from build123d import *
from build123d.topology import SkipClean

# Parameters (mm, degrees)
SKETCH_2_R                = 22
EXTRUDE_1_DEPTH           = 5
SKETCH_5_W                = 7
SKETCH_5_H                = 15
EXTRUDE_2_DEPTH           = 5
HOLE_WIZARD_2_56_3_D      = 1.778
HOLE_WIZARD_2_56_3_DEPTH  = 15
HOLE_WIZARD_2_56_3_TIP    = 0.534165
SKETCH_13_R               = 20.05
CUT_EXTRUDE_2_DEPTH       = 4
SKETCH_14_R               = 19
CUT_EXTRUDE_3_DEPTH       = 2
CUT_EXTRUDE_4_DEPTH       = 38.016888
EXTRUDE_3_REACH           = 58.225
EXTRUDE_3_END_RADIUS      = 22
SKETCH_16_W               = 18.5
SKETCH_16_H               = 5
FILLET_1_R                = 2
CHAMFER_1_SIZE            = 0.5
SKETCH_26_W               = 11.46
SKETCH_26_H               = 38.490745
CUT_EXTRUDE_5_DEPTH       = 38.138255
SKETCH_27_W               = 44
SKETCH_27_H               = 8
EXTRUDE_4_DEPTH           = 10
HOLE_WIZARD_2_D           = 4.5
HOLE_WIZARD_2_DEPTH       = 10.1
HOLE_WIZARD_2_CBORE_D     = 8
HOLE_WIZARD_2_CBORE_DEPTH = 4.6
HOLE_WIZARD_2_TIP         = 1.351936
EXTRUDE_5_DEPTH           = 5
EXTRUDE_6_REACH           = 60.062
EXTRUDE_6_END_RADIUS      = 22
SKETCH_32_W               = 5
SKETCH_32_H               = 22
MM_4_D                    = 2
MM_4_DEPTH                = 4
MM_4_TIP                  = 0.600861
SKETCH_41_R               = 2.2
CUT_EXTRUDE_6_DEPTH       = 3
SKETCH_45_W               = 27
SKETCH_45_H               = 5
EXTRUDE_7_DEPTH           = 2
EXTRUDE_9_REACH           = 62.756
SKETCH_47_W               = 10.54
SKETCH_47_H               = 5
HOLE_WIZARD_2_56_1_D      = 1.778
HOLE_WIZARD_2_56_1_DEPTH  = 5.73
HOLE_WIZARD_2_56_1_TIP    = 0.534165
FILLET_7_R                = 20
FILLET_8_R                = 5
HOLE_WIZARD_2_56_2_D      = 1.778
HOLE_WIZARD_M4_2_D        = 3.3
HOLE_WIZARD_M2_10_D       = 1.6


with BuildPart() as part:
    # 草图2 → 凸台-拉伸1 (new body)
    with BuildSketch(Plane.XY):
        Circle(SKETCH_2_R)
    extrude(amount=EXTRUDE_1_DEPTH)

    # 草图5 → 凸台-拉伸2 (add)
    with BuildSketch(Plane.XY.offset(5)):
        with Locations((0, 22)):
            Rectangle(SKETCH_5_W, SKETCH_5_H)
    extrude(amount=-EXTRUDE_2_DEPTH)

    # #2-56 螺纹孔3
    with Locations(Plane(origin=(0, 29.5, 2), x_dir=(0, 0, 1), z_dir=(0, 1, 0))):
        with Locations((0, 0)):
            Hole(HOLE_WIZARD_2_56_3_D / 2, depth=HOLE_WIZARD_2_56_3_DEPTH)
            with Locations((0, 0, -(HOLE_WIZARD_2_56_3_DEPTH + HOLE_WIZARD_2_56_3_TIP / 2))):  # 118° drill point
                Cone(0, HOLE_WIZARD_2_56_3_D / 2, HOLE_WIZARD_2_56_3_TIP, mode=Mode.SUBTRACT)

    # 草图13 → 切除-拉伸2 (cut)
    with BuildSketch(Plane(origin=(0, 0, 0), x_dir=(-1, 0, 0), z_dir=(0, 0, -1))):
        Circle(SKETCH_13_R)
    extrude(amount=-CUT_EXTRUDE_2_DEPTH, mode=Mode.SUBTRACT)

    # 草图14 → 切除-拉伸3 (cut)
    with BuildSketch(Plane(origin=(0, 0, 4), x_dir=(-1, 0, 0), z_dir=(0, 0, -1))):
        Circle(SKETCH_14_R)
    extrude(amount=-CUT_EXTRUDE_3_DEPTH, mode=Mode.SUBTRACT)

    # 草图15 → 切除-拉伸4 (cut, through all)
    with SkipClean():  # the faces are left unmerged after this step: merging them gives an invalid solid
        with BuildSketch(Plane(origin=(0, 0, 4), x_dir=(-1, 0, 0), z_dir=(0, 0, -1))):
            with BuildLine():
                Line((-10.630263, 17), (10.630263, 17))
                ThreePointArc((10.630263, 17), (20.05, 0), (10.630263, -17))
                Line((10.630263, -17), (-10.630263, -17))
                ThreePointArc((-10.630263, -17), (-20.05, 0), (-10.630263, 17))
            make_face()
        extrude(amount=-CUT_EXTRUDE_4_DEPTH, mode=Mode.SUBTRACT)

    # 凸台-拉伸3: up to this cylinder (the profile starts outside it)
    with SkipClean():  # the faces are left unmerged after this step: merging them gives an invalid solid
        extrude_3_end = Plane(origin=(0, 0, 2.5), z_dir=(0, 0, -1)) * Cylinder(EXTRUDE_3_END_RADIUS, 161.45, mode=Mode.PRIVATE)
        # 草图16 → 凸台-拉伸3 (add, up to the surface)
        with BuildSketch(Plane(origin=(0, 29.5, 0), x_dir=(1, 0, 0), z_dir=(0, 1, 0)), mode=Mode.PRIVATE) as extrude_3_sk1:
            with Locations((-12.75, -2.5)):
                Rectangle(SKETCH_16_W, SKETCH_16_H)
        extrude_3_tool1 = extrude(extrude_3_sk1.sketch, amount=-EXTRUDE_3_REACH, mode=Mode.PRIVATE) - extrude_3_end
        add(extrude_3_tool1.solids().sort_by_distance((-12.75, 29.5, 2.5))[0])
        # 草图16 → 凸台-拉伸3 (add, up to the surface)
        with BuildSketch(Plane(origin=(0, 29.5, 0), x_dir=(1, 0, 0), z_dir=(0, 1, 0)), mode=Mode.PRIVATE) as extrude_3_sk2:
            with Locations((12.75, -2.5)):
                Rectangle(SKETCH_16_W, SKETCH_16_H)
        extrude_3_tool2 = extrude(extrude_3_sk2.sketch, amount=-EXTRUDE_3_REACH, mode=Mode.PRIVATE) - extrude_3_end
        add(extrude_3_tool2.solids().sort_by_distance((12.75, 29.5, 2.5))[0])

    # 圆角1
    fillet_1_edges = [part.edges().sort_by_distance(p)[0] for p in [
        (8.485281, -17, 4.5),
        (-8.485281, -17, 4.5),
        (-8.485281, 17, 4.5),
        (8.485281, 17, 4.5),
        (10.630263, 17, 4.5),
        (10.630263, -17, 4.5),
    ]]
    fillet(fillet_1_edges, radius=FILLET_1_R)

    # 倒角1
    chamfer_1_edges = [part.edges().sort_by_distance(p)[0] for p in [
        (20.05, 0, 0),
    ]]
    chamfer(chamfer_1_edges, length=CHAMFER_1_SIZE)

    # 草图26 → 切除-拉伸5 (cut, through all)
    with SkipClean():  # the faces are left unmerged after this step: merging them gives an invalid solid
        with BuildSketch(Plane.XY.offset(5)):
            with Locations((-16.27, -2.245373)):
                Rectangle(SKETCH_26_W, SKETCH_26_H)
        extrude(amount=-CUT_EXTRUDE_5_DEPTH, mode=Mode.SUBTRACT)

    # 草图27 → 凸台-拉伸4 (add)
    with SkipClean():  # the faces are left unmerged after this step: merging them gives an invalid solid
        with BuildSketch(Plane(origin=(0, 0, 0), x_dir=(-1, 0, 0), z_dir=(0, 0, -1))):
            with Locations((0, 25.5)):
                Rectangle(SKETCH_27_W, SKETCH_27_H)
        extrude(amount=EXTRUDE_4_DEPTH)

    # 打孔尺寸(%根据)内六角圆柱头螺钉的类型2
    with Locations(Plane(origin=(-15, 21.5, -5), x_dir=(-1, 0, 0), z_dir=(0, -1, 0))):
        with Locations((0, 0), (-30, 0)):
            CounterBoreHole(HOLE_WIZARD_2_D / 2, HOLE_WIZARD_2_CBORE_D / 2, HOLE_WIZARD_2_CBORE_DEPTH, depth=HOLE_WIZARD_2_DEPTH)
            with Locations((0, 0, -(HOLE_WIZARD_2_DEPTH + HOLE_WIZARD_2_TIP / 2))):  # 118° drill point
                Cone(0, HOLE_WIZARD_2_D / 2, HOLE_WIZARD_2_TIP, mode=Mode.SUBTRACT)

    # 草图31 → 凸台-拉伸5 (add)
    with SkipClean():  # the faces are left unmerged after this step: merging them gives an invalid solid
        with BuildSketch(Plane(origin=(22, 0, 0), x_dir=(0, 0, -1), z_dir=(1, 0, 0))):
            Polygon((-5, 0), (0, 0), (0, 21.5), (10, 21.5), (10, 29.5), (-5, 29.5), align=None)
        extrude(amount=EXTRUDE_5_DEPTH)

    # 凸台-拉伸6: up to this cylinder (the profile starts outside it)
    with SkipClean():  # the faces are left unmerged after this step: merging them gives an invalid solid
        extrude_6_end = Plane(origin=(0, 0, 2.5), z_dir=(0, 0, -1)) * Cylinder(EXTRUDE_6_END_RADIUS, 165.124, mode=Mode.PRIVATE)
        # 草图32 → 凸台-拉伸6 (add, up to the surface)
        with BuildSketch(Plane(origin=(27, 0, 0), x_dir=(0, 0, -1), z_dir=(1, 0, 0)), mode=Mode.PRIVATE) as extrude_6_sk1:
            with Locations((-2.5, -11)):
                Rectangle(SKETCH_32_W, SKETCH_32_H)
        extrude_6_tool1 = extrude(extrude_6_sk1.sketch, amount=-EXTRUDE_6_REACH, mode=Mode.PRIVATE) - extrude_6_end
        add(extrude_6_tool1.solids().sort_by_distance((27, -11, 2.5))[0])

    # 大小mm 暗销孔4
    with Locations(Plane(origin=(-8, 29.5, -5), x_dir=(0, 0, 1), z_dir=(0, 1, 0))):
        with Locations((0, 0), (0, 16)):
            Hole(MM_4_D / 2, depth=MM_4_DEPTH)
            with Locations((0, 0, -(MM_4_DEPTH + MM_4_TIP / 2))):  # 118° drill point
                Cone(0, MM_4_D / 2, MM_4_TIP, mode=Mode.SUBTRACT)

    # 草图41 → 切除-拉伸6 (cut)
    with SkipClean():  # the faces are left unmerged after this step: merging them gives an invalid solid
        with BuildSketch(Plane(origin=(0, 29.5, 0), x_dir=(1, 0, 0), z_dir=(0, 1, 0))):
            with Locations(Location((0, -2, 0), (0, 0, 270))):
                Circle(SKETCH_41_R)
        extrude(amount=-CUT_EXTRUDE_6_DEPTH, mode=Mode.SUBTRACT)

    # 草图45 → 凸台-拉伸7 (add)
    with SkipClean():  # the faces are left unmerged after this step: merging them gives an invalid solid
        with BuildSketch(Plane.XZ.offset(22)):
            with Locations((13.5, 2.5)):
                Rectangle(SKETCH_45_W, SKETCH_45_H)
        extrude(amount=EXTRUDE_7_DEPTH)

    # 草图47 → 凸台-拉伸9 (add, up to next)
    with BuildSketch(Plane.XZ.offset(24), mode=Mode.PRIVATE) as extrude_9_sk1:
        with Locations((-5.27, 2.5)):
            Rectangle(SKETCH_47_W, SKETCH_47_H)
    extrude_9_tool1 = extrude(extrude_9_sk1.sketch, amount=-EXTRUDE_9_REACH, mode=Mode.PRIVATE) - part.part
    add(extrude_9_tool1.solids().sort_by_distance((-5.27, -24, 2.5))[0])

    # #2-56 螺纹孔1
    with Locations(Plane(origin=(0, -24, 2), x_dir=(0, 0, -1), z_dir=(0, -1, 0))):
        with Locations((0, 0)):
            Hole(HOLE_WIZARD_2_56_1_D / 2, depth=HOLE_WIZARD_2_56_1_DEPTH)
            with Locations((0, 0, -(HOLE_WIZARD_2_56_1_DEPTH + HOLE_WIZARD_2_56_1_TIP / 2))):  # 118° drill point
                Cone(0, HOLE_WIZARD_2_56_1_D / 2, HOLE_WIZARD_2_56_1_TIP, mode=Mode.SUBTRACT)

    # 圆角7
    # the kernel refuses this fillet: 20 mm, written as the material it takes off along each edge
    with BuildSketch(Plane(origin=(27, -24, -50), x_dir=(-1, 0, 0), z_dir=(0, 0, 1))) as fillet_7_piece_1:
        with BuildLine():
            CenterArc((FILLET_7_R, -FILLET_7_R), FILLET_7_R, 90, 90)
            Line((0, -FILLET_7_R), (0, 0))
            Line((0, 0), (FILLET_7_R, 0))
        make_face()
    extrude(amount=105, mode=Mode.SUBTRACT)

    # 圆角8
    # the kernel refuses this fillet: 5 mm, written as the material it takes off along each edge
    with BuildSketch(Plane(origin=(-10.54, -24, -12.5), x_dir=(0, 1, 0), z_dir=(0, 0, 1))) as fillet_8_piece_1:
        with BuildLine():
            CenterArc((FILLET_8_R, -FILLET_8_R), FILLET_8_R, 90, 90)
            Line((0, -FILLET_8_R), (0, 0))
            Line((0, 0), (FILLET_8_R, 0))
        make_face()
    extrude(amount=30, mode=Mode.SUBTRACT)

    # #2-56 螺纹孔2 (through all)
    with Locations(Plane(origin=(27, 0, 2), x_dir=(0, 0, 1), z_dir=(1, 0, 0))):
        with Locations((0, 0)):
            Hole(HOLE_WIZARD_2_56_2_D / 2)

    # M4 螺纹孔2 (through all)
    with Locations(Plane(origin=(0, 21.5, -6), x_dir=(-1, 0, 0), z_dir=(0, -1, 0))):
        with Locations((0, 0)):
            Hole(HOLE_WIZARD_M4_2_D / 2)

    # M2 螺纹孔10 (through all)
    with Locations(Plane(origin=(21.650635, 12.5, 0), x_dir=(-1, 0, 0), z_dir=(0, 0, -1))):
        with Locations((0, 0), (0, -25)):
            Hole(HOLE_WIZARD_M2_10_D / 2)


solid = part.part
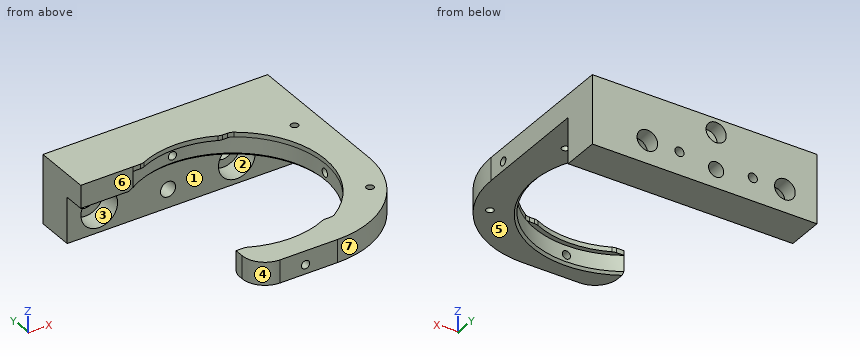
The listing builds one solid part. Answer for the finished solid, in the listing's coordinates (mm). Face numbers are marked on the shaded views. A direction names the side the tool comes from. Round coordinates to 2 decimals unless told otherwise and drop trailing zeros. Write each loop counter-clockwise with the first axis right and the second up, starting at its lowest first coordinate (ties: lowest second). Pieces come first, ordered by that corner, then holes. Notation, with made-up numbers: (29, 9) - (40, 9) arc R18 cw to (40, 41) - close; hole circle Ø5 at (-30, -0.5). An arc over 180 degrees is marked (long way). Use one line per item in the form item = value. Start each with the question number.
Item 1: A cutting plane is placed at B-B (x = 0). Give the number of separate pieces and of enclosed holes in the cut face, plus the area to 3 significant figures.
Item 2: Determine the mould class of the marked faces 1, 2, 3 and 4 for opening direction X: +X half, -X half, draft (parallel to the pull), parting line (faces both ways), or undercut.
Item 3: A tool of negligible diameter and unlimited length cuts with its end or side. For the marked faces 5, 6 and 7, from which of +Z, -Z, +X, -X, +Y, -Y can it reach the whole face along a straight path? Write none if from no direction.
Item 4: A cutting plane is placed at D-D (y = 0). Write down the section's boundary in (x, z).
Item 5: A cutting plane is placed at C-C (z = 2). Write down the section's boundary in (x, y), plus the area to 3 significant figures.
Item 6: Flat-ended cylindrical pins translate along their axes: pin 1 Ø1.1 at (x, z) = (9.5, 4.5) entering from -Y; pin 2 Ø0.8 at (x, z) = (-9.5, 4.5) entering from -Y; pin 3 Ø3 at (x, z) = (-8, -5) entering from +Y; pin 4 Ø6 at (y, z) = (17, -7) entering from +X. Find the tip coordinate at first contact, or state that the pin passes through.
Item 7: A cutting plane is placed at A-A (y = 23). Write down the section's boundary in (x, z), plus the area to 3 significant figures.
Item 8: Find the intervals of material crossed by line 1 (Z direction, x = 0, y = 24); line 2 (Z direction, x = 15, y = 28); line 3 (X direction, y = 28.1, z = 2), in increasing order. Write a range as [from, to].
The answers:
q1.separate_pieces = 5
q1.enclosed_holes = 0
q1.area = 90.8 mm^2
q2.face_1 = draft
q2.face_2 = undercut
q2.face_3 = undercut
q2.face_4 = -X half
q3.face_5 = -Z, +X, -X, -Y
q3.face_6 = +Z, -Z, -X, -Y
q3.face_7 = +Z, -Z, +X, -Y
q4.outline = (20.05, 0.5) - (20.55, 0) - (27, 0) - (27, 1.11) - (20.05, 1.11) - close; (20.05, 2.89) - (27, 2.89) - (27, 5) - (20.05, 5) - close
q5.outline = (-22, 17) - (-10.63, 17) arc R20.05 cw to (-0.89, 20.03) - (-0.89, 26.5) - (-2.2, 26.5) - (-2.2, 29.5) - (-22, 29.5) - close; (-10.54, -19) arc R5 ccw to (-5.54, -24) - (-0.89, -24) - (-0.89, -20.03) arc R20.05 cw to (-10.54, -17.06) - close; (0.89, -24) - (7, -24) arc R20 ccw to (27, -4) - (27, -0.89) - (20.03, -0.89) arc R20.05 cw to (0.89, -20.03) - close; (0.89, 20.03) arc R20.05 cw to (20.03, 0.89) - (27, 0.89) - (27, 29.5) - (2.2, 29.5) - (2.2, 26.5) - (0.89, 26.5) - close; hole circle Ø1.6 at (21.65, -12.5); hole circle Ø1.6 at (21.65, 12.5)
q5.area = 979 mm^2
q6.pin_1 = -23.9
q6.pin_2 = -22.51
q6.pin_3 = 29.5
q6.pin_4 = through
q7.outline = (-22, -10) - (27, -10) - (27, 5) - (-22, 5) - close; hole circle Ø8 at (-15, -5); hole circle Ø3.3 at (0, -6); hole circle Ø1.78 at (0, 2); hole circle Ø8 at (15, -5)
q7.area = 623 mm^2
q8.line_1 = [-10, -7.65], [-4.35, 1.11], [2.89, 5]
q8.line_2 = [-10, -7.25], [-2.75, 5]
q8.line_3 = [-22, -2.2], [2.2, 27]
